```python
from build123d import *

# Parameters (mm, degrees)
BOSS_EXTRUDE1_DEPTH = 300
SHELL1_T            = -10
FILLET1_R           = 30
FILLET2_R           = 10


with BuildPart() as part:
    # Sketch1 → Boss-Extrude1 (new body)
    with BuildSketch(Plane.XY):
        Polygon((-150, -16.621621622), (150, -16.621621622), (150, 83.378378378), (-150, 33.378378378), align=None)
    extrude(amount=BOSS_EXTRUDE1_DEPTH)

    # Shell1
    shell1_openings = [part.faces().sort_by_distance(p)[0] for p in [
        (0, 58.378378378, 150),
    ]]
    offset(amount=SHELL1_T, openings=shell1_openings, kind=Kind.INTERSECTION)

    # Fillet1
    fillet1_edges = [part.edges().sort_by_distance(p)[0] for p in [
        (150, 33.378378378, 300),
        (-150, 8.378378378, 300),
        (150, 33.378378378, 0),
        (-150, 8.378378378, 0),
    ]]
    fillet(fillet1_edges, radius=FILLET1_R)

    # Fillet2
    fillet2_edges = [part.edges().sort_by_distance(p)[0] for p in [
        (-140, 14.211711712, 10),
        (140, 37.545045045, 10),
        (-140, 14.211711712, 290),
        (140, 37.545045045, 290),
    ]]
    fillet(fillet2_edges, radius=FILLET2_R)


solid = part.part
```
Check sheet for the modelled part. Datum: model origin and axes. Units: mm. A direction names the side the tool comes from. Round coordinates to 2 decimals unless told otherwise and drop trailing zeros. Order: outer loops, then holes, each group sorted by start corner. A loop starts at its lowest first (then second) coordinate and runs counter-clockwise, first axis right, second up. Notation, with made-up numbers: (58, 37.5) - (106, 37.5) arc R16 ccw to (106, 46.5) - close; hole circle Ø6 at (67.25, 39.25). An arc over 180 degrees is marked (long way). Answer as CSV lines item,"result". Start each with the question number.
1) Section check D-D (y = 71). Record the cut outline in (x, z).
2) Draft check along Z on faces 1 (the face through (140, 37, 148)), 2 (the face through (-2, 21, 0)), 3 (the face through (141.445, 34.078, 290.979)). Enter one of: +Z half, -Z half, draft (parallel to the pull), parting line (faces both ways), or undercut.
3) Section check B-B (z = 141.5). Record the cut outline in (x, y), then the cut area to 3 significant figures.
4) Section check A-A (y = 23). Record the cut outline in (x, z), then the cut area to 3 significant figures.
5) Section check C-C (x = -17.5). Record the cut outline in (y, z).
6) Scan lines: probe 1 along Z at (x, y) = (-2.5, 7); probe 2 along X at (y, z) = (-0.5, 202); probe 3 along Y at (x, z) = (40, 272.5). Record each from-to range of solid material in increasing order.
7) Depth check by flat-ended pin: pin 1 (10 mm diameter, centred on x = 47, z = 261, fed in from +Y). Enter the tip coordinate at first touch or a pass-through.
8) Tool access check on faces 4 (the face through (137.15, 38.16, 13.01)), 5 (the face through (150, 33, 148)). Record the directions out of +Z, -Z, +X, -X, +Y, -Y that give a thin tool (end or side, any length) a straight path to the whole face; none if there is none.
Determined:
1,outline,"(75.73, 0) - (120, 0) arc R30 ccw to (150, 30) - (150, 270) arc R30 ccw to (120, 300) - (75.73, 300) - (75.73, 290) - (130, 290) arc R10 cw to (140, 280) - (140, 20) arc R10 cw to (130, 10) - (75.73, 10) - close"
2,face 1,"undercut"
2,face 2,"-Z half"
2,face 3,"+Z half"
3,outline,"(-150, -16.62) - (150, -16.62) - (150, 83.38) - (140, 81.71) - (140, -6.62) - (-140, -6.62) - (-140, 35.05) - (-150, 33.38) - close"
3,area,"4,300 mm^2"
4,outline,"(-150, 30) arc R30 ccw to (-120, 0) - (120, 0) arc R30 ccw to (150, 30) - (150, 270) arc R30 ccw to (120, 300) - (-120, 300) arc R30 ccw to (-150, 270) - close; hole (-140, 20) arc R10 ccw to (-130, 10) - (130, 10) arc R10 ccw to (140, 20) - (140, 280) arc R10 ccw to (130, 290) - (-130, 290) arc R10 ccw to (-140, 280) - close"
4,area,"10,900 mm^2"
5,outline,"(-16.62, 0) - (55.46, 0) - (55.46, 10) - (-6.62, 10) - (-6.62, 290) - (55.46, 290) - (55.46, 300) - (-16.62, 300) - close"
6,probe 1,"0 to 10, 290 to 300"
6,probe 2,"-150 to -140, 140 to 150"
6,probe 3,"-16.62 to -6.62"
7,pin 1,"y = -6.62"
8,face 4,"+Y"
8,face 5,"+Z, -Z, +X, +Y, -Y"
